Read the model definition and answer for the solid it produces. Units are mm, in the model's axes. A direction names the side the tool comes from. Coordinates: 2 decimals unless noted, no trailing zeros. Order: outer loops, then holes, each group sorted by start corner. A loop starts at its lowest first (then second) coordinate and runs counter-clockwise, first axis right, second up. Notation, with made-up numbers: (-2, 14) - (44, 14) arc R27 ccw to (44, 37) - close; hole circle Ø3 at (-24.5, 63). An arc over 180 degrees is marked (long way). Answer as a JSON object with one key per item and string values. Group by question number.
from build123d import *

# Parameters (mm, degrees)
EXTRUDE_1_DEPTH   = 10
EXTRUDE_1_2_DEPTH = 10
EXTRUDE_2_DEPTH   = 20
SKETCH_1_4_R      = 35
SKETCH_1_4_R_2    = 6
SKETCH_1_4_R_3    = 9
SKETCH_1_4_R_4    = 25
SKETCH_1_4_R_5    = 8
SKETCH_1_4_R_6    = 4
EXTRUDE_3_DEPTH   = 25


# Read off the part's stored shape, not the designer's step: the extrude step
with BuildPart() as part:
    # Sketch 1 → Extrude 1 (new body)
    with BuildSketch(Plane.XY):
        with BuildLine():
            ThreePointArc((-84.113248654, -80), (-87.773502692, -83.660254038), (-92.773502692, -85))
            Line((-92.773502692, -85), (-68.524791386, -85))
            Line((-68.524791386, -85), (-40.811978465, -85))
            ThreePointArc((-40.811978465, -85), (-54.668384925, -77), (-54.668384925, -61))
            Line((-54.668384925, -61), (-39.046205937, -33.941592266))
            ThreePointArc((-39.046205937, -33.941592266), (-30.151152872, -27.319125354), (-19.22989306, -29.243994476))
            ThreePointArc((-19.22989306, -29.243994476), (-32.622426184, -12.679799284), (-33.931812223, 8.580915992))
            ThreePointArc((-33.931812223, 8.580915992), (-34.876159455, 5.699155379), (-36.207821023, 2.974634616))
            Line((-36.207821023, 2.974634616), (-84.113248654, -80))
        make_face()
    extrude(amount=EXTRUDE_1_DEPTH)

    # Extrude 2 outline → Extrude 2 (add)
    with BuildSketch(Plane.XY):
        with BuildLine():
            ThreePointArc((91.622776602, -85), (83.171234054, -80.345224838), (82.587697573, -70.714285714))
            ThreePointArc((82.587697573, -70.714285714), (58.951595602, -84.978007291), (36.593908006, -68.783783784))
            ThreePointArc((36.593908006, -68.783783784), (35.222923087, -79.833937569), (25.358983849, -85))
            Line((25.358983849, -85), (-108.0001, -85))
            ThreePointArc((-108.0001, -85), (-118.606631007, -89.393368993), (-123, -99.9999))
            Line((-123, -99.9999), (115, -100))
            Line((115, -100), (115, -90))
            ThreePointArc((115, -90), (113.535533906, -86.464466094), (110, -85))
            Line((110, -85), (91.622776602, -85))
        make_face()
    extrude(amount=EXTRUDE_2_DEPTH)



with BuildPart() as body_2:
    # Sketch 1 → Extrude 1 2 (new body)
    with BuildSketch(Plane.XY):
        with BuildLine():
            ThreePointArc((33.089534913, -48.278298017), (35.418808442, -50.657512303), (35.737666875, -53.971800326))
            ThreePointArc((35.737666875, -53.971800326), (41.48802535, -43.198012184), (51.655818839, -36.433612056))
            ThreePointArc((51.655818839, -36.433612056), (34.49538534, -32.134623915), (31.785176497, -14.652732))
            ThreePointArc((31.785176497, -14.652732), (24.167277738, -25.316845908), (13.16091541, -32.431316741))
            ThreePointArc((13.16091541, -32.431316741), (16.80172204, -32.384616215), (19.508831427, -34.819613673))
            ThreePointArc((19.508831427, -34.819613673), (25.198282119, -42.659837887), (33.089534913, -48.278298017))
        make_face()
    extrude(amount=EXTRUDE_1_2_DEPTH)


with BuildPart() as part_1:
    add(part.part)

    add(body_2.part)  # Extrude 3 merges body 2
    # Sketch 1_4 → Extrude 3 (add)
    # profile 1 of 2: a face of its own
    with BuildSketch(Plane.XY):
        with Locations(Location((0, 0, 0), (0, 0, 165.808177005))):
            Circle(SKETCH_1_4_R)
        with Locations((-17.200292614, 13.716775641)):
            Circle(SKETCH_1_4_R_2, mode=Mode.SUBTRACT)
        with Locations((-21.448414068, -4.895460547)):
            Circle(SKETCH_1_4_R_2, mode=Mode.SUBTRACT)
        with Locations((-9.545442261, -19.821315094)):
            Circle(SKETCH_1_4_R_2, mode=Mode.SUBTRACT)
        with Locations((9.545442261, -19.821315094)):
            Circle(SKETCH_1_4_R_2, mode=Mode.SUBTRACT)
        with Locations((21.448414068, -4.895460547)):
            Circle(SKETCH_1_4_R_2, mode=Mode.SUBTRACT)
        with Locations((17.200292614, 13.716775641)):
            Circle(SKETCH_1_4_R_2, mode=Mode.SUBTRACT)
        with Locations((0, 22)):
            Circle(SKETCH_1_4_R_2, mode=Mode.SUBTRACT)
        Circle(SKETCH_1_4_R_3, mode=Mode.SUBTRACT)
    # profile 2 of 2: a face of its own
    with BuildSketch(Plane.XY):
        with Locations(Location((60, -60, 0), (0, 0, 166.046875379))):
            Circle(SKETCH_1_4_R_4)
        with Locations((60, -60)):
            Circle(SKETCH_1_4_R_5, mode=Mode.SUBTRACT)
        with Locations((45.277568136, -68.5)):
            Circle(SKETCH_1_4_R_6, mode=Mode.SUBTRACT)
        with Locations((74.722431864, -68.5)):
            Circle(SKETCH_1_4_R_6, mode=Mode.SUBTRACT)
        with Locations((60, -43)):
            Circle(SKETCH_1_4_R_6, mode=Mode.SUBTRACT)
    extrude(amount=EXTRUDE_3_DEPTH)


solid = part_1.part
1. Straight lines are drawn through the part: L1, parallel to Y at x = 0, z = 17; L2, parallel to Y at x = 18, z = 16.5; L3, parallel to X at y = 12, z = 23.5. For each, find the intervals that lie inside material, in ascending order.
2. For faces 1 (the cylindrical face through (35.399, -50.615, 4.93)), 2 (the cylindrical face through (-118.49, -89.28, 9.86)), 3 (the flat face through (31, -36, 10)), determine the directions among +Z, -Z, +X, -X, +Y, -Y from which every point of the face is accessible in a straight line to the end or side of a thin tool.
3. For a pull along Y with two mould halves and no side action, classify faces 4 (the flat face through (-6, -91, 20)), 5 (the cylindrical face through (114, -87, 10)), 6 (the cylindrical face through (25.1, -42.56, 4.93)) as pulls with the +Y half, pulls with the -Y half, needs draft (parallel to the pull), parting line crosses it, or undercut.
4. A cutting plane is placed at D-D on x = 94. Write down the section's boundary in (y, z), and give its area (3 significant figures).
5. Given pin 1 (19 mm diameter, centred on x = -9.55, y = -19.82, fed in from +Z); pin 2 (22 mm diameter, centred on x = -57.5, y = -31, fed in from +Z); pin 3 (4 mm diameter, centred on y = 13, z = 10.5, fed in from +X); pin 4 (8 mm diameter, centred on y = -53, z = 5, fed in from -X), each flat-ended and moving along its own axis, determine where each tip first touches the part or whether it passes through.
6. A cutting plane is placed at A-A on z = 14.75. State how many separate pieces and enclosed holes the cut face has, and give its area (3 significant figures).
7. A cutting plane is placed at B-B on y = -17. Write down the section's boundary in (x, z).
8. A cutting plane is placed at C-C on x = 0. Write down the section's boundary in (y, z), and give its area (3 significant figures).
Derived:
{
 "1": {"L1": "y = -100 to -85, -35 to -9, 9 to 16, 28 to 35", "L2": "y = -100 to -85, -30.02 to -9.81, 0.01 to 7.77, 19.66 to 30.02", "L3": "x = -32.88 to -22.95, -11.45 to 11.45, 22.95 to 32.88"},
 "2": {"face 1": "+Z, -Z", "face 2": "+Z, -Z, -X, +Y", "face 3": "+Z"},
 "3": {"face 4": "needs draft", "face 5": "pulls with the +Y half", "face 6": "undercut"},
 "4": {"outline": "(-100, 0) - (-85, 0) - (-85, 20) - (-100, 20) - close", "area": "300 mm2"},
 "5": {"pin 1": "stops at z = 25", "pin 2": "stops at z = 10", "pin 3": "stops at x = 33.23", "pin 4": "stops at x = -70.83"},
 "6": {"separate pieces": "2", "enclosed holes": "12", "area": "8,150 mm2"},
 "7": {"outline": "(-47.74, 0) - (-14.84, 0) - (-14.84, 25) - (-30.59, 25) - (-30.59, 10) - (-47.74, 10) - close; (-4.25, 0) - (4.25, 0) - (4.25, 25) - (-4.25, 25) - close; (14.84, 0) - (30.92, 0) - (30.92, 10) - (30.59, 10) - (30.59, 25) - (14.84, 25) - close"},
 "8": {"outline": "(-100, 0) - (-85, 0) - (-85, 20) - (-100, 20) - close; (-35, 0) - (-9, 0) - (-9, 25) - (-35, 25) - close; (9, 0) - (16, 0) - (16, 25) - (9, 25) - close; (28, 0) - (35, 0) - (35, 25) - (28, 25) - close", "area": "1,300 mm2"}
}
